Job drawing, mm, ordinate dimensions from the low corner. One solid piece. A direction names the side the tool comes from. Round coordinates to 2 decimals unless told otherwise and drop trailing zeros. Loops run counter-clockwise (first coordinate to the right, second up) from the corner with the lowest first, then second, coordinate; pieces in that order, holes last.
1) Band-saw the part on D-D, the plane y = 15.5. Write the cut outline in (x, z), then the cut area to 3 significant figures.
2) Probe line 1 (Y direction, x = 19, z = 4); line 2 (X direction, y = 6.25, z = 20); line 3 (Y direction, x = 28, z = 3.5). List the from-to ranges inside material, lowest first.
3) Band-saw the part on C-C, the plane z = 37.5. Write the cut outline in (x, y).
4) Drop flat-ended pins along their axis: P1, Ø1, axis at y = 17.5, z = 6.5, coming from the +X side; P2, Ø12, axis at x = 24, z = 19.5, coming from the +Y side; P3, Ø1.5, axis at x = 24, y = 18, coming from the +Z side; P4, Ø10, axis at y = 18.5, z = 27, coming from the +X side. Give the stop position or say it passes through.
5) 3-axis set-ups, long thin cutter, end or side, ignore diameter. For the marked faces 1 and 2: which of +Z, -Z, +X, -X, +Y, -Y reach the whole face in a straight line?
6) Mould opens along X. For the marked faces 3 and 4 say: +X half, -X half, draft (parallel to the pull), parting line (faces both ways), or undercut.
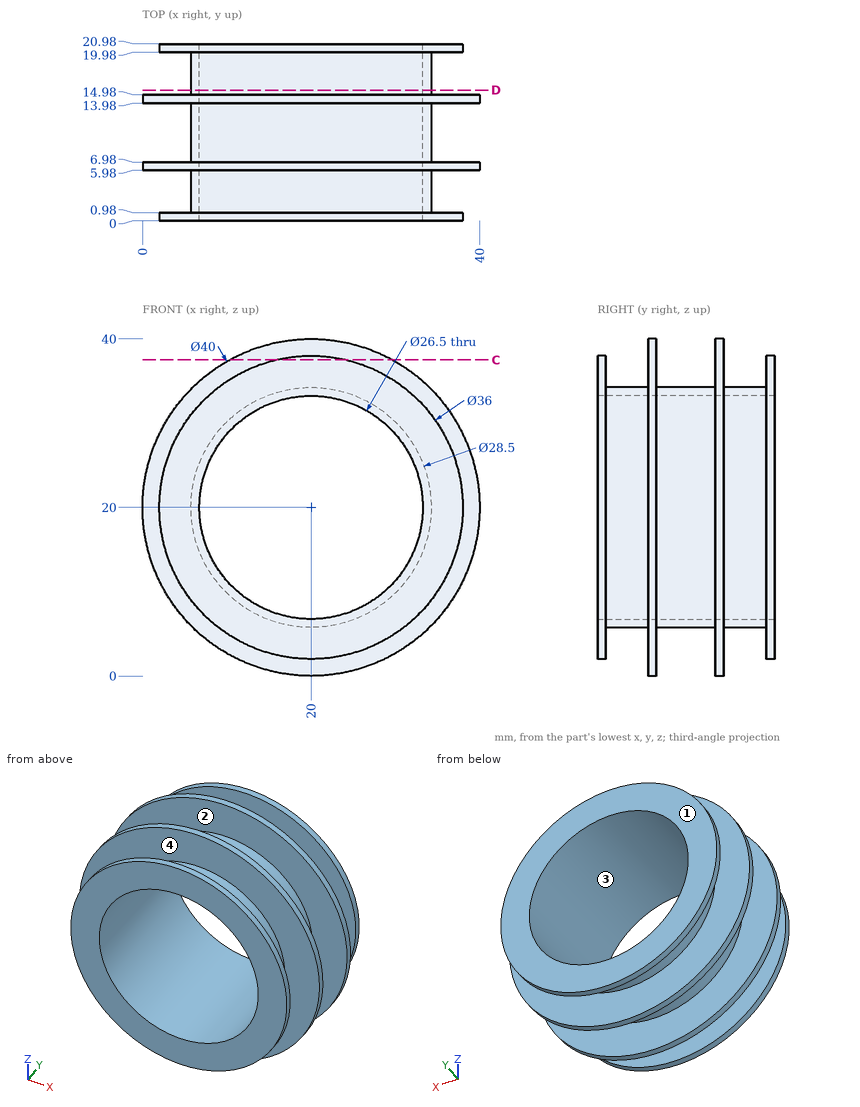
Reported:
1. outline: circle Ø28.5 at (20, 20); hole circle Ø26.5 at (20, 20)
1. area: 86.4 mm2
2. line 1: y = 0 to 0.98, 5.98 to 6.98, 13.98 to 14.98, 19.98 to 20.98
2. line 2: x = 0 to 6.75, 33.25 to 40
2. line 3: y = 5.98 to 6.98, 13.98 to 14.98
3. outline: (10.32, 5.98) - (29.68, 5.98) - (29.68, 6.98) - (10.32, 6.98) - close; (10.32, 13.98) - (29.68, 13.98) - (29.68, 14.98) - (10.32, 14.98) - close; (15.79, 0) - (24.21, 0) - (24.21, 0.98) - (15.79, 0.98) - close; (15.79, 19.98) - (24.21, 19.98) - (24.21, 20.98) - (15.79, 20.98) - close
4. P1: stops at x = 25.84
4. P2: passes through
4. P3: stops at z = 33.87
4. P4: stops at x = 39.7
5. face 1: +Z, -Z, +X, -X, +Y
5. face 2: none
6. face 3: undercut
6. face 4: draft
